Geometry: final body of the model. Coordinates: model frame, mm. Face numbers are marked on the shaded views. Round coordinates to 2 decimals unless told otherwise and drop trailing zeros. Order: outer loops, then holes, each group sorted by start corner. A loop starts at its lowest first (then second) coordinate and runs counter-clockwise, first axis right, second up. Notation, with made-up numbers: (89.5, 64) -> (100.5, 64) arc R28 ccw to (100.5, 87) -> close; hole circle Ø6 at (65, 34.5). An arc over 180 degrees is marked (long way). Put each result on its own line as item: value.
Autodesk Inventor part; units mm, degrees
ref_plane "Work Plane1" through (0, 0, 4.7) normal (0, 0, 1) x (1, 0, 0)
ref_plane "YZ Plane" through (0, 0, 0) normal (1, 0, 0) x (0, 1, 0)
ref_plane "XZ Plane" through (0, 0, 0) normal (0, 1, 0) x (-1, 0, 0)
sketch "Sketch1" plane through (0, 0, 0) normal (0, 0, 1) x (1, 0, 0)
  line L0 (-6.5078, 3.6754) -> (6.4922, 3.6754)
  line L1 (6.4922, 3.6754) -> (6.4922, -2.9246)
  line L2 (6.4922, -2.9246) -> (-6.5078, -2.9246)
  line L3 (-6.5078, -2.9246) -> (-6.5078, 3.6754)
  circle A0 centre (-3.5078, -2.0134) radius 0.5
  circle A1 centre (3.4922, -2.0134) radius 0.5
  point P0 (0, 0)
  dimension "d0" = 13
  dimension "d1" = 6.6
  dimension "d2" = 1
  dimension "d3" = 1
  dimension "d4" = 3
  dimension "d5" = 3
extrude "Extrusion1" add sketch "Sketch1" along normal blind 5.75
ref_plane "Work Plane1" through (0, 0, 4.7) normal (0, 0, 1) x (1, 0, 0)
sketch "Sketch2" plane through (0, 0, 4.7) normal (0, 0, 1) x (1, 0, 0)
  circle A0 centre (3.4922, -2.0134) radius 0.5
  circle A1 centre (-3.5078, -2.0134) radius 0.5
  line L0 (6.4922, 3.6754) -> (6.4922, -2.9246)
  line L1 (6.4922, -2.9246) -> (-6.5078, -2.9246)
  line L2 (-6.5078, -2.9246) -> (-6.5078, 3.6754)
  line L3 (-6.5078, 3.6754) -> (6.4922, 3.6754)
  line L4 (-5.5078, 3.6754) -> (-5.5078, 4.2754)
  line L5 (-5.2078, 3.6754) -> (-5.2078, 4.0146)
  line L6 (-5.2078, 4.0146) -> (7.6657, 5.8238)
  line L7 (-5.2078, 4.0146) -> (7.7922, 4.0146) construction
  line L8 (-5.5078, 4.2754) -> (7.624, 6.1209)
  line L9 (7.624, 6.1209) -> (7.6657, 5.8238)
  point P0 (0, 0)
  dimension "d9" = 0.6
  dimension "d10" = 0.3
  dimension "d11" = 1
  dimension "d12" = 13
  dimension "d13" = 8
  dimension "d14" = 0.3
extrude "Extrusion2" add sketch "Sketch2" against normal blind 3.6 contours L3 L4 L8 L9 L6 L5
sketch "Sketch3" plane through (-6.5078, -2.9246, 0) normal (0, -1, 0) x (1, 0, 0)
  line L0 (13, 0) -> (0, 0)
  line L1 (13, 0) -> (13, 5.75)
  line L2 (0, 5.75) -> (13, 5.75)
  line L3 (0, 0) -> (0, 5.75)
  line L4 (12.5, 2.2589) -> (11.5, 2.2589)
  line L5 (11.5, 2.2589) -> (11.5, 3.2589)
  line L6 (11.5, 3.2589) -> (12.5, 3.2589)
  line L7 (12.5, 3.2589) -> (12.5, 2.2589)
  line L8 (7, 2.2589) -> (6, 2.2589)
  line L9 (6, 2.2589) -> (6, 3.2589)
  line L10 (6, 3.2589) -> (7, 3.2589)
  line L11 (7, 3.2589) -> (7, 2.2589)
  line L12 (1.5, 2.2589) -> (0.5, 2.2589)
  line L13 (0.5, 2.2589) -> (0.5, 3.2589)
  line L14 (0.5, 3.2589) -> (1.5, 3.2589)
  line L15 (1.5, 3.2589) -> (1.5, 2.2589)
  point P0 (6.5078, 0)
  dimension "d17" = 1
  dimension "d18" = 1
  dimension "d19" = 0.5
  dimension "d22" = 5.5
extrude "Extrusion3" add sketch "Sketch3" along normal blind 4 contours L4 L5 L6 L7 | L8 L9 L10 L11 | L12 L13 L14 L15
fillet "Fillet1" radius 0.3 4 edges at (6.4922, 3.6754, 2.875) (6.4922, -2.9246, 2.875) (-6.5078, 3.6754, 2.875) (-6.5078, -2.9246, 2.875)
fillet "Fillet2" radius 0.3 2 edges at (-5.5078, 4.2754, 2.9) (-5.2078, 4.0146, 2.9)
equation "\"d5\" = d4"
equation "\"d14\" = d10"
properties part number "COTS_OMRON_D2FS-FL_Endstop"
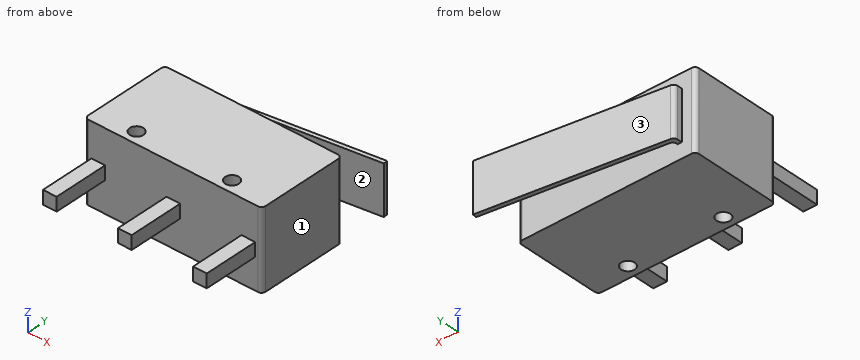
1. Cut plane B-B on z = 4.45. Return loops of the section in (x, y), and give its area (3 significant figures).
Ans:
outline: (-6.51, -2.62) arc R0.3 ccw to (-6.21, -2.92) -> (6.19, -2.92) arc R0.3 ccw to (6.49, -2.62) -> (6.49, 3.38) arc R0.3 ccw to (6.19, 3.68) -> (-5.21, 3.68) -> (-5.21, 3.75) arc R0.3 cw to (-4.95, 4.05) -> (7.67, 5.82) -> (7.62, 6.12) -> (-5.25, 4.31) arc R0.3 ccw to (-5.51, 4.01) -> (-5.51, 3.68) -> (-6.21, 3.68) arc R0.3 ccw to (-6.51, 3.38) -> close; hole circle Ø1 at (-3.51, -2.01); hole circle Ø1 at (3.49, -2.01)
area: 88.2 mm²
2. Contact query for flat-ended pins moving along their axis: P1, Ø1.1, axis at y = -5, z = 2.5, coming from the -X side; P2, Ø0.5, axis at y = -4.5, z = 3, coming from the +X side; P3, Ø1, axis at x = -5, z = 3, coming from the +Y side. Output: stop coordinate, or through.
Ans:
P1: x = -6.01
P2: x = 5.99
P3: y = 4.42
3. Cut plane C-C on x = -2.5. Return loops of the section in (y, z).
Ans:
outline: (-2.92, 0) -> (3.68, 0) -> (3.68, 5.75) -> (-2.92, 5.75) -> close; (4.4, 1.1) -> (4.7, 1.1) -> (4.7, 4.7) -> (4.4, 4.7) -> close
4. Cut plane A-A on y = -4.75. Return loops of the section in (x, z).
Ans:
outline: (-6.01, 2.26) -> (-5.01, 2.26) -> (-5.01, 3.26) -> (-6.01, 3.26) -> close; (-0.51, 2.26) -> (0.49, 2.26) -> (0.49, 3.26) -> (-0.51, 3.26) -> close; (4.99, 2.26) -> (5.99, 2.26) -> (5.99, 3.26) -> (4.99, 3.26) -> close
5. Cut plane D-D on y = 2.75. Return loops of the section in (x, z), and give its area (4 significant figures).
Ans:
outline: (-6.51, 0) -> (6.49, 0) -> (6.49, 5.75) -> (-6.51, 5.75) -> close
area: 74.75 mm²
6. Draft query along Y for the marked faces 1, 2 and 3. Return one class per face: +Y half, -Y half, draft (parallel to the pull), parting line (faces both ways), or undercut.
Ans:
face 1: draft
face 2: undercut
face 3: +Y half
7. Material intervals for probe 1 along Y at (x, z) = (3.5, 1.75); probe 2 along X at (y, z) = (0, 3.95); probe 3 along Y at (x, z) = (2.25, 2.8), sorted ascending.
Ans:
probe 1: -2.92 to -2.51, -1.51 to 3.68, 5.24 to 5.54
probe 2: -6.51 to 6.49
probe 3: -2.92 to 3.68, 5.06 to 5.37
